The model under review builds one solid part; all positions refer to its coordinate system, in mm. Coordinates: 2 decimals unless noted, no trailing zeros. Write each loop counter-clockwise with the first axis right and the second up, starting at its lowest first coordinate (ties: lowest second). Pieces come first, ordered by that corner, then holes.
1) Add section A-A, the plane z = 24. State the section outline as (x, y) points, then the cut area to 3 significant figures.
2) Add section B-B, the plane z = 33.5. State the section outline as (x, y) points.
3) Mouldability with a two-part tool opening along Y and no side actions: class faces 1 (the conical face through (2.48, 4.77, 6.91)), 2 (the flat face through (0, 4, 3.81)), 3 (the conical face through (20.206, -6.363, 5.582)) as released by +Y, released by -Y, zero draft, split by the parting line, or undercut.
4) For P1, Ø3, axis at x = 1.5, y = 7, coming from the -Z side; P2, Ø1.5, axis at y = -1.5, z = 32, coming from the +X side; P3, Ø8, axis at x = 5, z = 30.5, coming from the +Y side, all flat-tipped, find the tip position at first contact; note any pin that passes through.
5) For line 1 (Z direction, x = -17.5, y = 9.5); line 2 (Z direction, x = 7.5, y = -16.5); line 3 (Y direction, x = -8, z = 6), list the stretches that pass through material, from the lowest coordinate up.
from build123d import *


with BuildPart() as f1:
    # F0 (on Front) → F1 (revolve)
    with BuildSketch(Plane.XZ):
        with BuildLine():
            Line((1.178567, 38.1), (0, 38.1))
            Line((0, 38.1), (0, 0))
            Line((0, 0), (2.387992, 3.81))
            Line((2.387992, 3.81), (19.88674, 3.81))
            ThreePointArc((19.88674, 3.81), (20.769638, 4.167097), (21.156031, 5.037571))
            Line((21.156031, 5.037571), (21.315811, 8.169891))
            ThreePointArc((21.315811, 8.169891), (21.113608, 8.66767), (20.602155, 8.832246))
            Line((20.602155, 8.832246), (4.602036, 6.813674))
            ThreePointArc((4.602036, 6.813674), (4.11434, 6.95728), (3.888313, 7.412672))
            Line((3.888313, 7.412672), (3.626376, 12.770278))
            Line((3.626376, 12.770278), (2.447051, 36.892017))
            ThreePointArc((2.447051, 36.892017), (2.054391, 37.749691), (1.178567, 38.1))
        make_face()
    revolve(axis=Axis((0, 0, 19.05), (0, 0, -1)))


solid = f1.part
Geometry results:
1. outline: circle Ø6.15 at (0, 0)
1. area: 29.8 mm2
2. outline: circle Ø5.23 at (0, 0)
3. face 1: undercut
3. face 2: zero draft
3. face 3: split by the parting line
4. P1: stops at z = 3.81
4. P2: stops at x = 2.58
4. P3: stops at y = 2.59
5. line 1: z = 3.81 to 8.75
5. line 2: z = 3.81 to 8.52
5. line 3: y = -19.64 to 19.64
